Work out the finished part from the listing and answer in its coordinate system (mm). A direction names the side the tool comes from. Coordinates: 2 decimals unless noted, no trailing zeros. Loops run counter-clockwise (first coordinate to the right, second up) from the corner with the lowest first, then second, coordinate; pieces in that order, holes last. Notation, with made-up numbers: (-3.75, -10.75) -> (34.25, -10.75) arc R16 cw to (34.25, 5.25) -> close; hole circle Ø7 at (75, -5.75). An arc over 180 degrees is marked (long way). Answer as CSV lines item,"result".
Autodesk Inventor part; units mm, degrees
ref_plane "YZ Plane" through (0, 0, 0) normal (1, 0, 0) x (0, 1, 0)
ref_plane "XZ Plane" through (0, 0, 0) normal (0, 1, 0) x (-1, 0, 0)
ref_plane "XY Plane" through (0, 0, 0) normal (0, 0, 1) x (1, 0, 0)
sketch "Skizze1" plane through (0, 0, 0) normal (0, 0, 1) x (1, 0, 0)
  circle A0 centre (0, 0) radius 4.5
  dimension "d0" = 9
extrude "Extrusion1" add sketch "Skizze1" along normal blind 1
sketch "Skizze2" plane through (0, 0, 1) normal (0, 0, 1) x (1, 0, 0)
  circle A0 centre (0, 0) radius 4.5
  circle A1 centre (0, 0) radius 3.45
  dimension "d3" = 6.9
extrude "Extrusion2" add sketch "Skizze2" along normal blind 2.5 contours A1
chamfer "Fase2" distance 0.5 angle 45 1 edges at (-3.45, 0, 3.5)
properties part number "Servorückseitenlagerachse" material "Siliziumnitrid"
(1) Consider line 1 along Z through (x, y) = (3, 2.25); line 2 along X through (y, z) = (-2.75, 0.85); line 3 along X through (y, z) = (1, 3.1). Determine where each line is inside the solid, lowest interval first.
Computed values:
line 1,"0 to 1"
line 2,"-3.56 to 3.56"
line 3,"-3.2 to 3.2"
(2) A cutting plane is placed at C-C, the plane z = 3.25. Write down the section's boundary in (x, y).
Computed values:
outline,"circle Ø6.4 at (0, 0)"
(3) Flat-ended cylindrical pins translate along their axes: pin 1 Ø1.5 at (y, z) = (3.5, 1) entering from -X; pin 2 Ø2 at (y, z) = (-2, 0.5) entering from +X. Find the tip coordinate at first contact, or state that the pin passes through.
Computed values:
pin 1,"x = -3.56"
pin 2,"x = 4.39"
(4) A cutting plane is placed at A-A, the plane y = 0. Write down the section's boundary in (x, z), and give its area (3 significant figures).
Computed values:
outline,"(-4.5, 0) -> (4.5, 0) -> (4.5, 1) -> (3.45, 1) -> (3.45, 3) -> (2.95, 3.5) -> (-2.95, 3.5) -> (-3.45, 3) -> (-3.45, 1) -> (-4.5, 1) -> close"
area,"26.0 mm2"
(5) A cutting plane is placed at D-D, the plane z = 1.3. Write down the section's boundary in (x, y), and give its area (3 significant figures).
Computed values:
outline,"circle Ø6.9 at (0, 0)"
area,"37.4 mm2"
(6) Which of the six approach directions +Z, -Z, +X, -X, +Y, -Y give full straight-line access (tool end or side, diameter ignored) to faces 1 (the face through (0, 0, 0)), 2 (the face through (2, -3, 1))?
Computed values:
face 1,"-Z, +X, -X, +Y, -Y"
face 2,"+Z"
